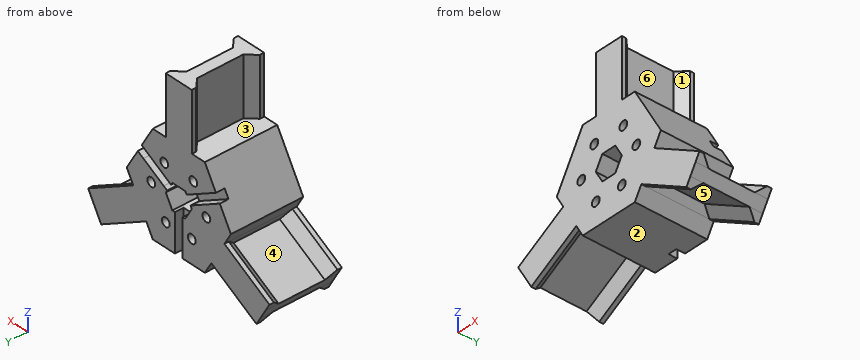
from build123d import *

# Parameters (mm, degrees)
SKETCH1_R           = 3
SKETCH1_W           = 6
SKETCH1_H           = 40
SKETCH1_W_2         = 8
BOSS_EXTRUDE1_DEPTH = 49.8
SKETCH1_4_W         = 6
SKETCH1_4_H         = 40
CUT_EXTRUDE2_DEPTH  = 46.8
SKETCH1_5_W         = 6
SKETCH1_5_H         = 40
BOSS_EXTRUDE3_DEPTH = 3
CHAMFER1_SIZE       = 6
SKETCH2_3_W         = 6
SKETCH2_3_H         = 17.980762113
SKETCH2_3_H_2       = 3
SKETCH2_3_H_3       = 5
CUT_EXTRUDE3_DEPTH  = 6


with BuildPart() as part:
    # Sketch1 → Boss-Extrude1 (new body)
    # profile 1 of 10: a face of its own
    with BuildSketch(Plane(origin=(0, 0, 0), x_dir=(1, 0, 0), z_dir=(0, 1, 0))):
        Polygon((20, -34.641016151), (40, 0), (20, 34.641016151), (-20, 34.641016151), (-40, 0), (-20, -34.641016151), align=None)
        with Locations(Location((21.160254038, -0.669872981, 0), (0, 0, 270))):
            Circle(SKETCH1_R, mode=Mode.SUBTRACT)
        with Locations(Location((10, 18.660254038, 0), (0, 0, 270))):
            Circle(SKETCH1_R, mode=Mode.SUBTRACT)
        with Locations(Location((-10, 18.660254038, 0), (0, 0, 270))):
            Circle(SKETCH1_R, mode=Mode.SUBTRACT)
        with Locations(Location((-21.160254038, -0.669872981, 0), (0, 0, 270))):
            Circle(SKETCH1_R, mode=Mode.SUBTRACT)
        with Locations(Location((11.160254038, -17.990381057, 0), (0, 0, 270))):
            Circle(SKETCH1_R, mode=Mode.SUBTRACT)
        with Locations(Location((-11.160254038, -17.990381057, 0), (0, 0, 270))):
            Circle(SKETCH1_R, mode=Mode.SUBTRACT)
        Polygon((10, 0), (5, 8.660254038), (-5, 8.660254038), (-10, 0), (-5, -8.660254038), (5, -8.660254038), align=None, mode=Mode.SUBTRACT)
    # profile 2 of 10: a face of its own
    with BuildSketch(Plane(origin=(0, 0, 0), x_dir=(1, 0, 0), z_dir=(0, 1, 0))):
        Polygon((-28, 20.784609691), (-25, 25.980762114), (-59.641016151, 45.980762114), (-62.641016151, 40.784609691), align=None)
    # profile 3 of 10: a face of its own
    with BuildSketch(Plane(origin=(0, 0, 0), x_dir=(1, 0, 0), z_dir=(0, 1, 0))):
        Polygon((-32, 13.856406461), (-28, 20.784609691), (-62.641016151, 40.784609691), (-66.641016151, 33.856406461), align=None)
    # profile 4 of 10: a face of its own
    with BuildSketch(Plane(origin=(0, 0, 0), x_dir=(1, 0, 0), z_dir=(0, 1, 0))):
        Polygon((-35, 8.660254038), (-32, 13.856406461), (-66.641016151, 33.856406461), (-69.641016151, 28.660254038), align=None)
    # profile 5 of 10: a face of its own
    with BuildSketch(Plane(origin=(0, 0, 0), x_dir=(1, 0, 0), z_dir=(0, 1, 0))):
        Polygon((59.641016151, 45.980762114), (25, 25.980762114), (28, 20.784609691), (62.641016151, 40.784609691), align=None)
    # profile 6 of 10: a face of its own
    with BuildSketch(Plane(origin=(0, 0, 0), x_dir=(1, 0, 0), z_dir=(0, 1, 0))):
        Polygon((62.641016151, 40.784609691), (28, 20.784609691), (32, 13.856406461), (66.641016151, 33.856406461), align=None)
    # profile 7 of 10: a face of its own
    with BuildSketch(Plane(origin=(0, 0, 0), x_dir=(1, 0, 0), z_dir=(0, 1, 0))):
        Polygon((66.641016151, 33.856406461), (32, 13.856406461), (35, 8.660254038), (69.641016151, 28.660254038), align=None)
    # profile 8 of 10: a face of its own
    with BuildSketch(Plane(origin=(0, 0, 0), x_dir=(1, 0, 0), z_dir=(0, 1, 0))):
        with Locations((7, -54.641016151)):
            Rectangle(SKETCH1_W, SKETCH1_H)
    # profile 9 of 10: a face of its own
    with BuildSketch(Plane(origin=(0, 0, 0), x_dir=(1, 0, 0), z_dir=(0, 1, 0))):
        with Locations((-7, -54.641016151)):
            Rectangle(SKETCH1_W, SKETCH1_H)
    # profile 10 of 10: a face of its own
    with BuildSketch(Plane(origin=(0, 0, 0), x_dir=(1, 0, 0), z_dir=(0, 1, 0))):
        with Locations((0, -54.641016151)):
            Rectangle(SKETCH1_W_2, SKETCH1_H)
    extrude(amount=BOSS_EXTRUDE1_DEPTH)

    # Sketch1<4> → Cut-Extrude2 (cut)
    with BuildSketch(Plane(origin=(0, 0, 0), x_dir=(1, 0, 0), z_dir=(0, 1, 0))):
        Polygon((59.641016151, 45.980762114), (25, 25.980762114), (28, 20.784609691), (62.641016151, 40.784609691), align=None)
        Polygon((-28, 20.784609691), (-25, 25.980762114), (-59.641016151, 45.980762114), (-62.641016151, 40.784609691), align=None)
        Polygon((66.641016151, 33.856406461), (32, 13.856406461), (35, 8.660254038), (69.641016151, 28.660254038), align=None)
        Polygon((-35, 8.660254038), (-32, 13.856406461), (-66.641016151, 33.856406461), (-69.641016151, 28.660254038), align=None)
        with Locations((7, -54.641016151)):
            Rectangle(SKETCH1_4_W, SKETCH1_4_H)
        with Locations((-7, -54.641016151)):
            Rectangle(SKETCH1_4_W, SKETCH1_4_H)
    extrude(amount=CUT_EXTRUDE2_DEPTH, mode=Mode.SUBTRACT)

    # Sketch1<5> → Boss-Extrude3 (add)
    with BuildSketch(Plane(origin=(0, 0, 0), x_dir=(1, 0, 0), z_dir=(0, 1, 0))):
        with Locations((-7, -54.641016151)):
            Rectangle(SKETCH1_5_W, SKETCH1_5_H)
        with Locations((7, -54.641016151)):
            Rectangle(SKETCH1_5_W, SKETCH1_5_H)
        Polygon((-35, 8.660254038), (-32, 13.856406461), (-66.641016151, 33.856406461), (-69.641016151, 28.660254038), align=None)
        Polygon((-28, 20.784609691), (-25, 25.980762114), (-59.641016151, 45.980762114), (-62.641016151, 40.784609691), align=None)
        Polygon((66.641016151, 33.856406461), (32, 13.856406461), (35, 8.660254038), (69.641016151, 28.660254038), align=None)
        Polygon((59.641016151, 45.980762114), (25, 25.980762114), (28, 20.784609691), (62.641016151, 40.784609691), align=None)
    extrude(amount=BOSS_EXTRUDE3_DEPTH)

    # Chamfer1
    chamfer1_edges = [part.edges().sort_by_distance(p)[0] for p in [
        (-45.320508076, 46.8, -30.784609691),
        (-45.320508076, 3, -30.784609691),
        (-49.320508076, 46.8, -23.856406461),
        (-49.320508076, 3, -23.856406461),
        (49.320508076, 46.8, -23.856406461),
        (45.320508076, 46.8, -30.784609691),
        (45.320508076, 3, -30.784609691),
        (49.320508076, 3, -23.856406461),
        (-4, 3, 54.641016151),
        (4, 3, 54.641016151),
        (4, 46.8, 54.641016151),
        (-4, 46.8, 54.641016151),
    ]]
    chamfer(chamfer1_edges, length=CHAMFER1_SIZE - 0.0001)  # a hair under: the kernel refuses the full size

    # Sketch2<3> → Cut-Extrude3 (cut)
    with BuildSketch(Plane(origin=(0, 49.8, 0), x_dir=(1, 0, 0), z_dir=(0, 1, 0))):
        Polygon((-24.169872981, -17.418584287), (-27.169872981, -12.222431864), (-31.5, -14.722431864), (-28.5, -19.918584287), align=None)
        Polygon((-9, -1.732050808), (-11.598076211, -3.232050808), (-8.598076211, -8.42820323), (-6, -6.92820323), align=None)
        Polygon((8.598076211, -8.42820323), (11.598076211, -3.232050808), (9, -1.732050808), (6, -6.92820323), align=None)
        Polygon((31.5, -14.722431864), (27.169872981, -12.222431864), (24.169872981, -17.418584287), (28.5, -19.918584287), align=None)
        Polygon((27.169872981, -12.222431864), (11.598076211, -3.232050808), (8.598076211, -8.42820323), (24.169872981, -17.418584287), align=None)
        Polygon((-11.598076211, -3.232050808), (-27.169872981, -12.222431864), (-24.169872981, -17.418584287), (-8.598076211, -8.42820323), align=None)
        with Locations((0, 20.650635095)):
            Rectangle(SKETCH2_3_W, SKETCH2_3_H)
        with Locations((0, 10.160254038)):
            Rectangle(SKETCH2_3_W, SKETCH2_3_H_2)
        with Locations((0, 32.141016151)):
            Rectangle(SKETCH2_3_W, SKETCH2_3_H_3)
    extrude(amount=-CUT_EXTRUDE3_DEPTH, mode=Mode.SUBTRACT)


solid = part.part
The listing builds one solid part. Answer for the finished solid, in the listing's coordinates (mm). Face numbers are marked on the shaded views. A direction names the side the tool comes from. Give positions to 0.01 mm unless a question says otherwise; leave off trailing zeros. One line per item, written item: value. Start each with the question number.
1) A tool of negligible diameter and unlimited length cuts with its end or side. For the marked faces 4, 5 and 6, from which of +Z, -Z, +X, -X, +Y, -Y can it reach the whole face along a straight path? Write none if from no direction.
2) Find the intervals of material crossed by L1, parallel to X at y = 41, z = -25; L2, parallel to X at y = 39, z = -27.5; L3, parallel to Z at x = 12, y = 24, in increasing order.
3) Given pin 1 Ø10 at (x, y) = (19.5, 11) entering from -Z; pin 2 Ø10 at (y, z) = (20.5, 17) entering from -X; pin 3 Ø3 at (y, z) = (40, 43) entering from +X; pin 4 Ø12 at (x, z) = (-39, 17) entering from +Y, each flat-ended and moving along its own axis, determine where each tip first touches the part or whether it passes through.
4) The mould has two halves that part along X. Classify the marked faces 1, 2 and 3: released by +X, released by -X, zero draft, split by the parting line, or undercut.
5) A cutting plane is placed at C-C on y = 19.5. State how many separate pieces and enclosed holes the cut face has, then the cut area to 3 significant figures.
Answer sheet:
1. face 4: -X
1. face 5: -Z
1. face 6: +Z, +X
2. L1: x = -51.7 to -34.9, -25.57 to 25.57, 34.9 to 51.7
2. L2: x = -55.63 to -39.63, -24.12 to 24.12, 39.63 to 55.63
2. L3: z = -34.64 to -20.9, -16.42 to 15.11, 20.87 to 34.64
3. pin 1: stops at z = -34.64
3. pin 2: stops at x = -33.07
3. pin 3: stops at x = 4.7
3. pin 4: passes through
4. face 1: released by +X
4. face 2: undercut
4. face 3: zero draft
5. separate pieces: 1
5. enclosed holes: 7
5. area: 4,690 mm2
